```python
from build123d import *

# Parameters (mm, degrees)
ESQUISSE1_W             = 25
ESQUISSE1_H             = 40
BOSS_EXTRU_1_DEPTH      = 6
ESQUISSE2_R             = 1.005
ENL_V_MAT_EXTRU_1_DEPTH = 6
ESQUISSE3_R             = 2
ENL_V_MAT_EXTRU_2_DEPTH = 3
ESQUISSE4_W             = 7.5
ESQUISSE4_H             = 6
BOSS_EXTRU_2_DEPTH      = 6


with BuildPart() as part:
    # Esquisse1 → Boss.-Extru.1 (new body)
    with BuildSketch(Plane.XY):
        with Locations((12.5, 20)):
            Rectangle(ESQUISSE1_W, ESQUISSE1_H)
    extrude(amount=BOSS_EXTRU_1_DEPTH)

    # Esquisse2 → Enlèv. mat.-Extru.1 (cut)
    with BuildSketch(Plane.XY.offset(6)):
        with Locations((4.5, 37)):
            Circle(ESQUISSE2_R)
        with Locations((20.5, 37)):
            Circle(ESQUISSE2_R)
        with Locations((4.5, 21)):
            Circle(ESQUISSE2_R)
        with Locations((20.5, 21)):
            Circle(ESQUISSE2_R)
    extrude(amount=-ENL_V_MAT_EXTRU_1_DEPTH, mode=Mode.SUBTRACT)

    # Esquisse3 → Enlèv. mat.-Extru.2 (cut)
    with BuildSketch(Plane.XY.offset(6)):
        with Locations((4.5, 37)):
            Circle(ESQUISSE3_R)
        with Locations((20.5, 37)):
            Circle(ESQUISSE3_R)
        with Locations((4.5, 21)):
            Circle(ESQUISSE3_R)
        with Locations((20.5, 21)):
            Circle(ESQUISSE3_R)
    extrude(amount=-ENL_V_MAT_EXTRU_2_DEPTH, mode=Mode.SUBTRACT)

    # Esquisse4 → Boss.-Extru.2 (add)
    with BuildSketch(Plane.XZ):
        with Locations((3.75, 3)):
            Rectangle(ESQUISSE4_W, ESQUISSE4_H)
        with Locations((21.25, 3)):
            Rectangle(ESQUISSE4_W, ESQUISSE4_H)
    extrude(amount=BOSS_EXTRU_2_DEPTH)


solid = part.part
```
Geometry: final body of the model. Coordinates: model frame, mm. A direction names the side the tool comes from. Coordinates: 2 decimals unless noted, no trailing zeros. Order: outer loops, then holes, each group sorted by start corner. A loop starts at its lowest first (then second) coordinate and runs counter-clockwise, first axis right, second up. Notation, with made-up numbers: (-21.5, 46) -> (33.5, 46) arc R23 ccw to (33.5, 81) -> close; hole circle Ø11 at (-8, -38.5). An arc over 180 degrees is marked (long way). Write item = value, one per line.
(1) Cut plane D-D on z = 3.6. Return loops of the section in (x, y), plus the area to 3 significant figures.
Solved:
outline = (0, -6) -> (7.5, -6) -> (7.5, 0) -> (17.5, 0) -> (17.5, -6) -> (25, -6) -> (25, 40) -> (0, 40) -> close; hole circle Ø4 at (4.5, 21); hole circle Ø4 at (4.5, 37); hole circle Ø4 at (20.5, 21); hole circle Ø4 at (20.5, 37)
area = 1,040 mm²
(2) Cut plane A-A on x = 20.5. Return loops of the section in (y, z) (3 decimals), plus the area to 3 significant figures.
Solved:
outline = (-6, 0) -> (19.995, 0) -> (19.995, 3) -> (19, 3) -> (19, 6) -> (-6, 6) -> close; (22.005, 0) -> (35.995, 0) -> (35.995, 3) -> (35, 3) -> (35, 6) -> (23, 6) -> (23, 3) -> (22.005, 3) -> close; (38.005, 0) -> (40, 0) -> (40, 6) -> (39, 6) -> (39, 3) -> (38.005, 3) -> close
area = 240 mm²
(3) Cut plane B-B on y = 37. Return loops of the section in (x, z) (3 decimals), plus the area to 3 significant figures.
Solved:
outline = (0, 0) -> (3.495, 0) -> (3.495, 3) -> (2.5, 3) -> (2.5, 6) -> (0, 6) -> close; (5.505, 0) -> (19.495, 0) -> (19.495, 3) -> (18.5, 3) -> (18.5, 6) -> (6.5, 6) -> (6.5, 3) -> (5.505, 3) -> close; (21.505, 0) -> (25, 0) -> (25, 6) -> (22.5, 6) -> (22.5, 3) -> (21.505, 3) -> close
area = 114 mm²
(4) Pin query (flat end, axial travel): pin 1 Ø3 at (x, y) = (20.5, 21) entering from -Z; pin 2 Ø3 at (x, y) = (4.5, 37) entering from +Z. Return the tip coordinate at first contact, or that it passes through.
Solved:
pin_1 = 0
pin_2 = 3
(5) Access query for faces 1 (the cylindrical face through (19.026, 22.352, 4.521)), 2 (the flat face through (12, 0, 3)), 3 (the flat face through (12, 17, 0)). Directions: +Z, -Z, +X, -X, +Y, -Y. A direction counts if a zero-diameter tool reaches every point of the face in a straight line with its end or side. Return the directions, or none.
Solved:
face_1 = +Z
face_2 = +Z, -Z, -Y
face_3 = -Z, +X, -X, +Y, -Y
(6) Pull-direction query (X, two-part tool) for faces 4 (the flat face through (21, -6, 3)), 5 (the flat face through (25, 17, 3)), 6 (the flat face through (21.4, 20.1, 3)), 7 (the flat face through (7.5, -3, 3)); classes: pulls with the +X half, pulls with the -X half, needs draft (parallel to the pull), parting line crosses it, or undercut.
Solved:
face_4 = needs draft
face_5 = pulls with the +X half
face_6 = undercut
face_7 = undercut
(7) Line query: line 1 (Y direction, x = 20.5, z = 0.9) (3 decimals); line 2 (Y direction, x = 4.5, z = 5.25); line 3 (X direction, y = -1.5, z = 2.2). Output: solid intervals per line, ascending.
Solved:
line_1 = -6 to 19.995, 22.005 to 35.995, 38.005 to 40
line_2 = -6 to 19, 23 to 35, 39 to 40
line_3 = 0 to 7.5, 17.5 to 25
(8) Cut plane C-C on y = -2. Return loops of the section in (x, z).
Solved:
outline = (0, 0) -> (7.5, 0) -> (7.5, 6) -> (0, 6) -> close; (17.5, 0) -> (25, 0) -> (25, 6) -> (17.5, 6) -> close
